Here's how the part is built. I have some questions about the finished solid (model axes, mm). A direction names the side the tool comes from. Round coordinates to 2 decimals unless told otherwise and drop trailing zeros. Write each loop counter-clockwise with the first axis right and the second up, starting at its lowest first coordinate (ties: lowest second). Pieces come first, ordered by that corner, then holes. Notation, with made-up numbers: (-38, 47.25) -> (-29, 47.25) arc R22 ccw to (-29, 86.25) -> close; hole circle Ø2 at (25.5, 12). An arc over 180 degrees is marked (long way). Answer in a Markdown table with one row per item.
from build123d import *

# Parameters (mm, degrees)
F1_DEPTH  = 11
F2_W      = 8
F2_H      = 45
F2_W_2    = 8.5
F2_H_2    = 15
F3_DEPTH  = 25
F4_R      = 7.49999
F5_R      = 10.99999
F6_R      = 7.99999
F7_R      = 2
F8_R      = 3
F9_DEPTH  = 19
F10_R     = 3
F11_DEPTH = 35
F12_SIZE  = 0.5


# Not quite as in the source:
# - a fillet or chamfer is up to 0.001 mm smaller than in the source, because OpenCascade refuses the exact size


with BuildPart() as f1:
    # F0 (on Front) → F1 (new body, symmetric)
    with BuildSketch(Plane.XZ):
        Polygon((-15, -11), (0, -11), (0, 0), (8.5, 0), (8.5, 20), (22.5, 20), (22.5, 28), (8.5, 28), (8.5, 40), (22.5, 40), (22.5, 48), (-2.5, 48), (-2.5, 40), (0.5, 40), (0.5, 8), (-18.5, 8), (-18.5, 0), (-15, 0), align=None)
    extrude(amount=F1_DEPTH, both=True)

    # F2 (on Right) → F3 (cut, symmetric)
    with BuildSketch(Plane.YZ):
        with Locations((-12, 30.5)):
            Rectangle(F2_W, F2_H)
        with Locations((12, 30.5)):
            Rectangle(F2_W, F2_H)
        with Locations((-11.75, -7.5)):
            Rectangle(F2_W_2, F2_H_2)
        with Locations((11.75, -7.5)):
            Rectangle(F2_W_2, F2_H_2)
    extrude(amount=F3_DEPTH, both=True, mode=Mode.SUBTRACT)

    # F4 (radius 7.5 in the source; OpenCascade refuses exactly that, so slightly less here)
    f4_edges = [f1.edges().sort_by_distance(p)[0] for p in [
        (0, -7.5, -5.5),
        (-15, -7.5, -5.5),
        (0, 7.5, -5.5),
        (-15, 7.5, -5.5),
    ]]
    fillet(f4_edges, radius=F4_R)

    # F5 (radius 11 in the source; OpenCascade refuses exactly that, so slightly less here)
    f5_edges = [f1.edges().sort_by_distance(p)[0] for p in [
        (-18.5, 11, 4),
        (-18.5, -11, 4),
    ]]
    fillet(f5_edges, radius=F5_R)

    # F6 (radius 8 in the source; OpenCascade refuses exactly that, so slightly less here)
    f6_edges = [f1.edges().sort_by_distance(p)[0] for p in [
        (22.5, 8, 44),
        (22.5, 8, 24),
        (22.5, -8, 24),
        (22.5, -8, 44),
    ]]
    fillet(f6_edges, radius=F6_R)

    # F7
    f7_edges = [f1.edges().sort_by_distance(p)[0] for p in [
        (8.5, 0, 28),
        (8.5, 0, 40),
        (0.5, 0, 40),
        (0.5, 0, 8),
        (4.5, -8, 8),
        (4.5, 8, 8),
        (8.5, 0, 20),
    ]]
    fillet(f7_edges, radius=F7_R)

    # F8 (on face) → F9 (cut)
    with BuildSketch(Plane.XY.offset(8)):
        with Locations((-7.5, 0)):
            Circle(F8_R)
    extrude(amount=-F9_DEPTH, mode=Mode.SUBTRACT)

    # F10 (on face) → F11 (cut)
    with BuildSketch(Plane.XY.offset(48)):
        with Locations((14.5, 0)):
            Circle(F10_R)
    extrude(amount=-F11_DEPTH, mode=Mode.SUBTRACT)

    # F12
    f12_edges = [f1.edges().sort_by_distance(p)[0] for p in [
        (-12.803304, -5.303304, -11),
    ]]
    chamfer(f12_edges, length=F12_SIZE)


solid = f1.part
1) I want a section at B-B, the plane x = 12.5. List the corners of the cut face in (y, z) for me.
Response:
| item | result |
|---|---|
| outline | (-8, 20) -> (-2.24, 20) -> (-2.24, 28) -> (-8, 28) -> close; (-8, 40) -> (-2.24, 40) -> (-2.24, 48) -> (-8, 48) -> close; (2.24, 20) -> (8, 20) -> (8, 28) -> (2.24, 28) -> close; (2.24, 40) -> (8, 40) -> (8, 48) -> (2.24, 48) -> close |
2) Which directions (+Z, -Z, +X, -X, +Y, -Y) give clear straight access to the entire face, cutting with the end or side of a thin tool? Please do faces 4 (the face through (6, -8, 29)), 5 (the face through (0.5, 0, 24)), 6 (the face through (-12.745, 5.361, -5.324)), 7 (the face through (18, 0, 28)).
Response:
| item | result |
|---|---|
| face 4 | +Z, +X, -X, -Y |
| face 5 | -X, +Y, -Y |
| face 6 | -Z, -X, +Y |
| face 7 | +X, +Y, -Y |
3) I want a section at C-C, the plane z = 31.5. List the corners of the cut face in (x, y) for me, and give its area (3 significant figures).
Response:
| item | result |
|---|---|
| outline | (0.5, -8) -> (8.5, -8) -> (8.5, 8) -> (0.5, 8) -> close |
| area | 128 mm^2 |
4) For pin 1 (4 mm diameter, centred on y = 2.5, z = 6, fed in from +X); pin 2 (2.5 mm diameter, centred on y = -1.5, z = 44.5, fed in from -X); pin 3 (12 mm diameter, centred on y = -3.5, z = 34.5, fed in from +X), each with a flat end and sliding along its axis, tell me the tip position at first contact or that it passes through.
Response:
| item | result |
|---|---|
| pin 1 | stops at x = 8.5 |
| pin 2 | stops at x = -2.5 |
| pin 3 | stops at x = 22.42 |
5) We'd pull the mould along Z, two halves only. Please class faces 1 (the face through (8.5, 0, 34)), 2 (the face through (9.07, -0.11, 19.4)), 3 (the face through (11.5, 0.1, 44.1)): +Z half, -Z half, draft (parallel to the pull), parting line (faces both ways), or undercut.
Response:
| item | result |
|---|---|
| face 1 | undercut |
| face 2 | -Z half |
| face 3 | draft |
6) I need wall thicknesses on line 1 (Y direction, x = 14.5, z = 22); line 2 (Z direction, x = -2, y = 3.75); line 3 (Z direction, x = 13, y = -5.5). Which ranges of each line are inside material? Lowest first, please. Write a range as [from, to].
Response:
| item | result |
|---|---|
| line 1 | y = [-8, -3], [3, 8] |
| line 2 | z = [-11, 8], [40, 48] |
| line 3 | z = [20, 28], [40, 48] |
